from build123d import *

# Parameters (mm, degrees)
BOSS_EXTRUDE1_DEPTH = 10
FILLET3_R           = 3
SKETCH1_3_W         = 5
SKETCH1_3_H         = 1.5
BOSS_EXTRUDE2_DEPTH = 30
BOSS_EXTRUDE3_DEPTH = 2.5
FILLET1_R           = 2.5
FILLET4_R           = 0.1


with BuildPart() as part:
    # Sketch1 → Boss-Extrude1 (new body)
    with BuildSketch(Plane(origin=(0, 0, 0), x_dir=(1, 0, 0), z_dir=(0, 1, 0))):
        with BuildLine():
            ThreePointArc((2.545584412, 3.15), (0, -4.05), (-2.545584412, 3.15))
            Line((-2.545584412, 3.15), (-4.2, 3.15))
            ThreePointArc((-4.2, 3.15), (-5.128577821, -1.122581638), (-2.5, -4.616546328))
            Line((-2.5, -4.616546328), (-2.5, -6.816546328))
            Line((-2.5, -6.816546328), (2.5, -6.816546328))
            Line((2.5, -6.816546328), (2.5, -4.616546328))
            ThreePointArc((2.5, -4.616546328), (5.128577821, -1.122581638), (4.2, 3.15))
            Line((4.2, 3.15), (2.545584412, 3.15))
        make_face()
    extrude(amount=BOSS_EXTRUDE1_DEPTH)

    # Fillet3
    fillet3_edges = [part.edges().sort_by_distance(p)[0] for p in [
        (-2.5, 5, 4.616546328),
        (2.5, 5, 4.616546328),
    ]]
    fillet(fillet3_edges, radius=FILLET3_R)

    # Sketch1<3> → Boss-Extrude2 (add)
    with BuildSketch(Plane(origin=(0, 0, 0), x_dir=(1, 0, 0), z_dir=(0, 1, 0))):
        with Locations((0, -6.066546328)):
            Rectangle(SKETCH1_3_W, SKETCH1_3_H)
    extrude(amount=BOSS_EXTRUDE2_DEPTH)

    # Sketch2 → Boss-Extrude3 (add, symmetric)
    with BuildSketch(Plane.ZY):
        with BuildLine():
            Line((5.316546328, 25.10300567), (5.316546328, 30))
            ThreePointArc((5.316546328, 30), (4.05, 27.551502835), (5.316546328, 25.10300567))
        make_face()
    extrude(amount=BOSS_EXTRUDE3_DEPTH, both=True)

    # Fillet1
    fillet1_edges = [part.edges().sort_by_distance(p)[0] for p in [
        (0, 30, 5.316546328),
        (0, 25.10300567, 5.316546328),
    ]]
    fillet(fillet1_edges, radius=FILLET1_R)

    # Fillet4
    fillet4_edges = [part.edges().sort_by_distance(p)[0] for p in [
        (-4.2, 5, -3.15),
        (-2.545584412, 5, -3.15),
        (2.545584412, 5, -3.15),
        (4.2, 5, -3.15),
    ]]
    fillet(fillet4_edges, radius=FILLET4_R)


solid = part.part
Can you work these out from the model? Positions are in its coordinate system, mm. A direction names the side the tool comes from. Coordinates: 2 decimals unless noted, no trailing zeros. Order: outer loops, then holes, each group sorted by start corner. A loop starts at its lowest first (then second) coordinate and runs counter-clockwise, first axis right, second up. Notation, with made-up numbers: M 69,8 L 102,8 A24 ccw 102,31 Z; hole C 39,-25 d10. An arc over 180 degrees is marked long. Answer as CSV lines item,"result".
(1) Suppose I cut it at B-B on x = 0. Please give me the cut outline in (y, z), plus the area to 3 significant figures.
Geometry check:
outline,"M 0,4.05 L 10,4.05 L 10,5.32 L 24.04,5.32 A2.5 cw 25.64,4.74 A3 ccw 27.24,4.07 A2.5 ccw 30,6.55 L 30,6.82 L 0,6.82 Z"
area,"61.7 mm^2"
(2) On a 3-axis mill with a long thin cutter (end or side, diameter ignored), from which of +Z, -Z, +X, -X, +Y, -Y can I reach the whole of each face in a straight line? I mean faces 4 (the flat face through (0, 17, 5.317)), 5 (the flat face through (2.5, 19, 6)), 6 (the flat face through (0, 15, 6.817)). Say none if no direction works.
Geometry check:
face 4,"-Z, +X, -X"
face 5,"+Z, +X, +Y"
face 6,"+Z, +X, -X, +Y, -Y"
(3) I'm going to push flat-ended pins straight in: pin 1 (4 mm diameter, centred on x = -1, y = 19.5, fed in from -Z); pin 2 (2 mm diameter, centred on y = 14.5, z = 5, fed in from +X); pin 3 (3 mm diameter, centred on x = -1.5, z = 3, fed in from +Y). Where does each tip first touch, or does it pass through?
Geometry check:
pin 1,"z = 5.32"
pin 2,"x = 2.5"
pin 3,"y = 28.93"
(4) Suppose I cut it at D-D on z = -2.25. Please give me the cut outline in (x, y), plus the area to 3 significant figures.
Geometry check:
outline,"M -4.74,0 L -3.37,0 L -3.37,10 L -4.74,10 Z; M 3.37,0 L 4.74,0 L 4.74,10 L 3.37,10 Z"
area,"27.5 mm^2"
(5) Please list where these lines run through material, in increasing order: L1, parallel to X at y = 5.75, z = 0; L2, parallel to Z at x = 0, y = 7.75; L3, parallel to Z at x = 2, y = 21.5.
Geometry check:
L1,"-5.25 to -4.05, 4.05 to 5.25"
L2,"4.05 to 6.82"
L3,"5.32 to 6.82"
(6) Suppose I cut it at A-A on z = 0. Please give me the cut outline in (x, y), plus the area to 3 significant figures.
Geometry check:
outline,"M -5.25,0 L -4.05,0 L -4.05,10 L -5.25,10 Z; M 4.05,0 L 5.25,0 L 5.25,10 L 4.05,10 Z"
area,"24.0 mm^2"
(7) Suppose I cut it at C-C on y = 8.25. Please give me the cut outline in (x, z), plus the area to 3 significant figures.
Geometry check:
outline,"M -4.23,-3.11 A0.1 ccw -4.15,-3.15 L -2.81,-3.15 A0.1 ccw -2.75,-2.98 A4.05 cw long 2.75,-2.98 A0.1 ccw 2.81,-3.15 L 4.15,-3.15 A0.1 ccw 4.23,-3.11 A5.25 ccw 3.5,3.91 A3 cw 2.5,6.15 L 2.5,6.82 L -2.5,6.82 L -2.5,6.15 A3 cw -3.5,3.91 A5.25 ccw Z"
area,"35.3 mm^2"
(8) If we mould it in two halves opening along X, with no side actions, what happens to faces 1 (the cylindrical face through (2.754, 5.07, 4.941)), 2 (the flat face through (-2.5, 19, 6)), 3 (the cylindrical face through (0.136, 4.93, 4.048))? For each: released by +X, released by -X, zero draft, split by the parting line, or undercut.
Geometry check:
face 1,"released by +X"
face 2,"released by -X"
face 3,"undercut"
